```python
from build123d import *

# Parameters (mm, degrees)
BOSS_EXTRUDE1_DEPTH = 7.5
CHAMFER1_SIZE       = 2.5
SKETCH2_R           = 16.5
BOSS_EXTRUDE2_DEPTH = 5
BOSS_EXTRUDE3_START = -5
BOSS_EXTRUDE3_DEPTH = 5
SKETCH4_R           = 5
CUT_EXTRUDE1_DEPTH  = 10
SKETCH5_R           = 5
BOSS_EXTRUDE4_DEPTH = 10


with BuildPart() as part:
    # Sketch1 → Boss-Extrude1 (new, symmetric)
    with BuildSketch(Plane.XY):
        with BuildLine():
            ThreePointArc((169.186105477, 14.977902914), (85.617423728, 13.934366249), (2.253460208, 19.872642429))
            ThreePointArc((2.253460208, 19.872642429), (-19.801791361, 2.808746854), (-3.361833105, -19.715427415))
            ThreePointArc((-3.361833105, -19.715427415), (85.256800738, -25.931146508), (173.369675456, -14.61660998))
            ThreePointArc((173.369675456, -14.61660998), (184.852333231, 2.099570811), (169.186105477, 14.977902914))
        make_face()
    extrude(amount=BOSS_EXTRUDE1_DEPTH, both=True)

    # Chamfer1
    chamfer1_edges = [part.edges().sort_by_distance(p)[0] for p in [
        (85.617423728, 13.934366249, 7.5),
        (184.852333231, 2.099570811, 7.5),
        (184.852333231, 2.099570811, -7.5),
        (-19.801791361, 2.808746854, 7.5),
        (85.256800738, -25.931146508, 7.5),
        (-19.801791361, 2.808746854, -7.5),
        (85.617423728, 13.934366249, -7.5),
        (85.256800738, -25.931146508, -7.5),
    ]]
    chamfer(chamfer1_edges, length=CHAMFER1_SIZE)

    # Sketch2 → Boss-Extrude2 (add)
    with BuildSketch(Plane.XY.offset(7.5)):
        Circle(SKETCH2_R)
    extrude(amount=BOSS_EXTRUDE2_DEPTH)

    # Sketch3 → Boss-Extrude3 (add)
    with BuildSketch(Plane.XY.offset(12.5).offset(BOSS_EXTRUDE3_START)):
        with BuildLine():
            ThreePointArc((-0.253915773, 19.358335376), (-2.55345676, 18.462340064), (-3.403051231, 16.145254483))
            ThreePointArc((-3.403051231, 16.145254483), (0.863543278, 16.477387323), (5.0720476, 15.701093374))
            ThreePointArc((5.0720476, 15.701093374), (4.469308692, 18.094292522), (2.276021844, 19.225746964))
            Line((2.276021844, 19.225746964), (-0.253915773, 19.358335376))
        make_face()
        with BuildLine():
            ThreePointArc((14.30344882, 8.225652062), (15.249383609, 6.301293481), (15.937776134, 4.270514244))
            Line((15.937776134, 4.270514244), (18.660254038, 5))
            Line((18.660254038, 5), (18.332406715, 6.223542865))
            ThreePointArc((18.332406715, 6.223542865), (16.76966729, 8.133658527), (14.30344882, 8.225652062))
        make_face()
        with BuildLine():
            Line((18.660254038, 5), (15.937776134, 4.270514244))
            ThreePointArc((15.937776134, 4.270514244), (16.357000338, 2.167611574), (16.499976071, 0.028100762))
            ThreePointArc((16.499976071, 0.028100762), (18.58978715, 1.340878735), (18.98810136, 3.776457135))
            Line((18.98810136, 3.776457135), (18.660254038, 5))
        make_face()
        with BuildLine():
            ThreePointArc((11.583966219, -15.511974356), (12.917681126, -13.435462641), (12.243068758, -11.061521929))
            ThreePointArc((12.243068758, -11.061521929), (8.986544078, -13.838064371), (5.125498425, -15.683726148))
            ThreePointArc((5.125498425, -15.683726148), (7.01981161, -17.265583889), (9.459270178, -16.891768097))
            Line((9.459270178, -16.891768097), (11.583966219, -15.511974356))
        make_face()
        with BuildLine():
            ThreePointArc((-11.173121868, -15.810470249), (-8.786101299, -16.437231094), (-6.736816201, -15.062048582))
            ThreePointArc((-6.736816201, -15.062048582), (-10.383786452, -12.822908364), (-13.332243835, -9.721176591))
            ThreePointArc((-13.332243835, -9.721176591), (-14.25130498, -12.011596414), (-13.141950881, -14.21614395))
            Line((-13.141950881, -14.21614395), (-11.173121868, -15.810470249))
        make_face()
        with BuildLine():
            Line((0, 0), (-13.017345465, 9.457655082))
            ThreePointArc((-13.017345465, 9.457655082), (-15.632747256, 9.907063304), (-17.581442501, 8.105707948))
            Line((-17.581442501, 8.105707948), (-18.489335293, 5.740566364))
            ThreePointArc((-18.489335293, 5.740566364), (-18.246514507, 3.097966821), (-16.002179404, 1.681896829))
            Line((-16.002179404, 1.681896829), (0, 0))
        make_face()
    extrude(amount=BOSS_EXTRUDE3_DEPTH)

    # Sketch4 → Cut-Extrude1 (cut)
    with BuildSketch(Plane.XY.offset(7.5)):
        with Locations((170, 0)):
            Circle(SKETCH4_R)
    extrude(amount=-CUT_EXTRUDE1_DEPTH, mode=Mode.SUBTRACT)

    # Sketch5 → Boss-Extrude4 (add)
    with BuildSketch(Plane(origin=(0, 0, -7.5), x_dir=(-1, 0, 0), z_dir=(0, 0, -1))):
        with Locations(Location((0, 0, 0), (0, 0, 180))):
            Circle(SKETCH5_R)
    extrude(amount=BOSS_EXTRUDE4_DEPTH)


solid = part.part
```
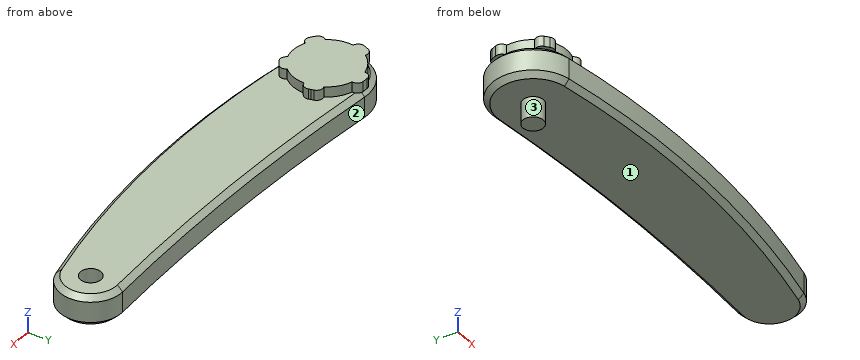
Work out the finished part from the listing and answer in its coordinate system (mm). Face numbers are marked on the shaded views. Give positions to 0.01 mm unless a question says otherwise; leave off trailing zeros. Write each loop counter-clockwise with the first axis right and the second up, starting at its lowest first coordinate (ties: lowest second). Pieces come first, ordered by that corner, then holes.
(1) The part is cut by section B-B on z = -12.25. Write down the section's boundary in (x, y), plus the area to 3 significant figures.
Final values:
outline: circle Ø10 at (0, 0)
area: 78.5 mm2
(2) Straight lines are drawn through the part: line 1 (Z direction, x = 77.5, y = -8); line 2 (Y direction, x = 170, z = 4); line 3 (Z direction, x = 15.5, y = 2). For each, find the intervals that lie inside material, in ascending order.
Final values:
line 1: z = -7.5 to 7.5
line 2: y = -15.38 to -5, 5 to 15
line 3: z = -7.5 to 12.5
(3) Flat-ended cylindrical pins translate along their axes: pin 1 Ø20.5 at (x, y) = (81, -5) entering from +Z; pin 2 Ø1.9 at (x, y) = (1, 18.5) entering from -Z; pin 3 Ø12.5 at (x, y) = (105.5, 2) entering from -Z. Find the tip coordinate at first contact, or state that the pin passes through.
Final values:
pin 1: stops at z = 7.5
pin 2: stops at z = -7.42
pin 3: stops at z = -7.5
(4) The mould has two halves that part along X. Classify the marked faces 1, 2 and 3: pulls with the +X half, pulls with the -X half, needs draft (parallel to the pull), parting line crosses it, or undercut.
Final values:
face 1: needs draft
face 2: undercut
face 3: parting line crosses it
(5) The part is cut by section A-A on z = 3.25. Write down the section's boundary in (x, y), plus the area to 3 significant figures.
Final values:
outline: (-3.36, -19.72) arc R450 ccw to (173.37, -14.62) arc R15 ccw to (169.19, 14.98) arc R1000 cw to (2.25, 19.87) arc R20 ccw to start; hole circle Ø10 at (170, 0)
area: 7,430 mm2
